Build history of the part. All positions in model axes, mm. Round coordinates to 2 decimals unless told otherwise and drop trailing zeros. Write each loop counter-clockwise with the first axis right and the second up, starting at its lowest first coordinate (ties: lowest second). Pieces come first, ordered by that corner, then holes. Notation, with made-up numbers: M -38.5,21.25 L 10.5,21.25 A9 ccw 10.5,32.25 Z; hole C 79,-26 d5. An arc over 180 degrees is marked long. Write item = value, one per line.
Autodesk Inventor part; units mm, degrees
ref_plane "YZ Plane" through (0, 0, 0) normal (1, 0, 0) x (0, 1, 0)
ref_plane "XZ Plane" through (0, 0, 0) normal (0, 1, 0) x (-1, 0, 0)
ref_plane "XY Plane" through (0, 0, 0) normal (0, 0, 1) x (1, 0, 0)
sketch "Sketch1" plane through (0, 0, 0) normal (0, 1, 0) x (-1, 0, 0)
  line L0 (0, 25.4) -> (25.4, 25.4)
  line L1 (25.4, 25.4) -> (25.4, 0)
  line L2 (25.4, 0) -> (0, 0)
  line L3 (0, 0) -> (0, 25.4)
  line L4 (22.225, 22.225) -> (3.175, 22.225)
  line L5 (3.175, 22.225) -> (3.175, 3.175)
  line L6 (3.175, 3.175) -> (22.225, 3.175)
  line L7 (22.225, 3.175) -> (22.225, 22.225)
  dimension "d0" = 25.4
  dimension "d1" = 25.4
  dimension "d2" = 3.175
extrude "Extrusion1" add sketch "Sketch1" along normal blind 609.6
sketch "Sketch2" plane through (-25.4, 0, 25.4) normal (0, 0, 1) x (1, 0, 0)
  circle A0 centre (12.7, 491.5841) radius 3.302
  circle A1 centre (12.7, 452.2611) radius 3.302
  circle A2 centre (12.7, 412.9381) radius 3.302
  circle A3 centre (12.7, 373.6152) radius 3.302
  circle A4 centre (12.7, 334.2922) radius 3.302
  circle A5 centre (12.7, 294.9693) radius 3.302
  circle A6 centre (12.7, 255.6463) radius 3.302
  circle A7 centre (12.7, 216.3233) radius 3.302
  circle A8 centre (12.7, 177.0004) radius 3.302
  circle A9 centre (12.7, 137.6774) radius 3.302
  circle A10 centre (12.7, 98.3544) radius 3.302
  circle A11 centre (12.7, 118.0159) radius 3.302
  circle A12 centre (12.7, 157.3389) radius 3.302
  circle A13 centre (12.7, 196.6619) radius 3.302
  circle A14 centre (12.7, 235.9848) radius 3.302
  circle A15 centre (12.7, 275.3078) radius 3.302
  circle A16 centre (12.7, 314.6307) radius 3.302
  circle A17 centre (12.7, 353.9537) radius 3.302
  circle A18 centre (12.7, 393.2767) radius 3.302
  circle A19 centre (12.7, 432.5996) radius 3.302
  circle A20 centre (12.7, 471.9226) radius 3.302
  circle A21 centre (12.7, 511.2456) radius 3.302
  line L0 (0, 25.4) -> (25.4, 25.4)
  line L1 (0, 25.4) -> (0, 584.2)
  line L2 (25.4, 584.2) -> (0, 584.2)
  line L3 (25.4, 25.4) -> (25.4, 584.2)
extrude "Extrusion2" cut sketch "Sketch2" against normal through all contours A0 | A1 | A2 | A3 | A4 | A5 | A6 | A7 | A8 | A9 | A10 | A11 | A12 | A13 | A14 | A15 | A16 | A17 | A18 | A19 | A20 | A21
sketch "Sketch3" plane through (-25.4, 0, 0) normal (-1, 0, 0) x (0, 0, 1)
  line L0 (25.4, 0) -> (25.4, 609.6)
  line L1 (0, 0) -> (0, 609.6)
  line L2 (0, 511.2456) -> (25.4, 511.2456) construction
  line L3 (0, 373.6152) -> (25.4, 373.6152) construction
  line L4 (0, 235.9848) -> (25.4, 235.9848) construction
  line L5 (0, 98.3544) -> (25.4, 98.3544) construction
  line L6 (12.7, 523.9456) -> (12.7, 479.4956) construction
  line L7 (12.7, 403.7777) -> (12.7, 343.4527) construction
  line L8 (12.7, 258.2098) -> (12.7, 213.7598) construction
  line L9 (12.7, 130.1044) -> (12.7, 85.6544) construction
  circle A0 centre (12.7, 523.9456) radius 3.302
  circle A1 centre (12.7, 479.4956) radius 3.302
  circle A2 centre (12.7, 403.7777) radius 3.302
  circle A3 centre (12.7, 343.4527) radius 3.302
  circle A4 centre (12.7, 258.2098) radius 3.302
  circle A5 centre (12.7, 213.7598) radius 3.302
  circle A6 centre (12.7, 130.1044) radius 3.302
  circle A7 centre (12.7, 85.6544) radius 3.302
  line L10 (0, 304.8) -> (25.4, 304.8) construction
  line L11 (12.7, 334.9625) -> (12.7, 274.6375) construction
  circle A8 centre (12.7, 334.9625) radius 3.302
  circle A9 centre (12.7, 274.6375) radius 3.302
  line L12 (0, 609.6) -> (25.4, 609.6)
  line L13 (0, 107.8794) -> (25.4, 107.8794) construction
  line L14 (25.4, 0) -> (0, 0)
  circle A10 centre (12.7, 596.9) radius 3.302
  circle A11 centre (12.7, 574.675) radius 3.302
  circle A12 centre (12.7, 558.8) radius 3.302
  line L15 (0, 501.7206) -> (25.4, 501.7206) construction
  circle A13 centre (12.7, 12.7) radius 3.302
  circle A14 centre (12.7, 34.925) radius 3.302
  circle A15 centre (12.7, 50.8) radius 3.302
  line L16 (22.225, 507.9436) -> (22.225, 514.5476)
  line L17 (22.225, 95.0524) -> (22.225, 101.6564)
  line L18 (22.225, 232.6828) -> (22.225, 239.2868)
  line L19 (22.225, 370.3132) -> (22.225, 376.9172)
  point P0 (12.7, 235.9848)
  point P1 (12.7, 373.6152)
  point P2 (12.7, 304.8)
  point P3 (12.7, 107.8794)
  point P4 (12.7, 501.7206)
  point P5 (22.225, 511.2456)
  point P6 (22.225, 373.6152)
  point P7 (22.225, 235.9848)
  point P8 (22.225, 98.3544)
  dimension "d7" = 44.45
  dimension "d8" = 60.325
  dimension "d9" = 44.45
  dimension "d10" = 44.45
  dimension "d11" = 6.604
  dimension "d12" = 6.604
  dimension "d13" = 6.604
  dimension "d14" = 6.604
  dimension "d15" = 6.604
  dimension "d16" = 6.604
  dimension "d17" = 6.604
  dimension "d18" = 6.604
  dimension "d21" = 60.325
  dimension "d22" = 6.604
  dimension "d23" = 6.604
  dimension "d27" = 9.525
  dimension "d28" = 9.525
extrude "Extrusion3" cut sketch "Sketch3" against normal blind 25.4 contours A0 | A1 | A6 | A7 | A8 | A9 | A10 | A11 | A12 | A13 | A14 | A15
equation "\"d9\" = d7"
equation "\"d10\" = d7"
equation "\"d12\" = d11"
equation "\"d13\" = d11"
equation "\"d14\" = d11"
equation "\"d15\" = d11"
equation "\"d16\" = d11"
equation "\"d17\" = d11"
equation "\"d18\" = d11"
equation "\"d21\" = d8"
equation "\"d22\" = d11"
equation "\"d23\" = d11"
equation "\"d27\" = d28"
properties part number "Chassis V1.500 Part1" material "Aluminum 6061"
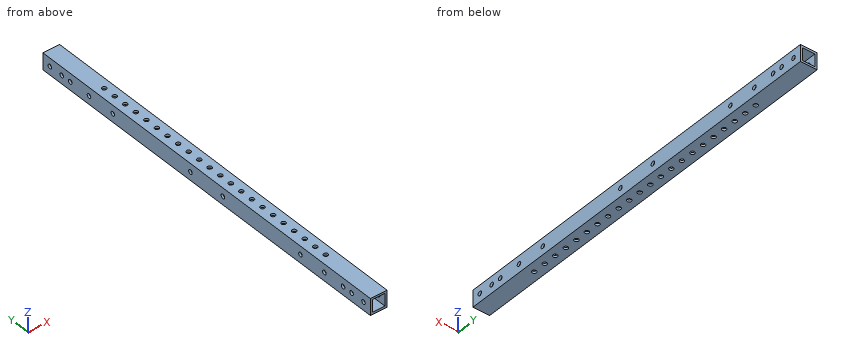
1. Flat gauge pin, fed straight in: pin 1 (4 mm diameter, centred on y = 574.675, z = 12.7, fed in from +X). Where does the tip first touch, or does it go through?
Responses:
pin_1 = through
2. Band-saw the part on A-A (y = 384). List the corners of the cut face in (x, z) (3 decimals), plus the area to 3 significant figures.
Responses:
outline = M -25.4,0 L 0,0 L 0,25.4 L -25.4,25.4 Z; hole M -22.225,3.175 L -3.175,3.175 L -3.175,22.225 L -22.225,22.225 Z
area = 282 mm²
3. Probe probe 1 along X at (y, z) = (355, 5) (3 decimals); probe 2 along Z at (x, y) = (-8, 393.5) (3 decimals); probe 3 along X at (y, z) = (372, 2). List the from-to ranges inside material, lowest first.
Responses:
probe_1 = -25.4 to -22.225, -3.175 to 0
probe_2 = 0 to 3.175, 22.225 to 25.4
probe_3 = -25.4 to -15.58, -9.82 to 0
